Model file for the job. Use its own axes, mm. Give positions to 0.01 mm unless a question says otherwise; leave off trailing zeros. Loops run counter-clockwise (first coordinate to the right, second up) from the corner with the lowest first, then second, coordinate; pieces in that order, holes last. Notation, with made-up numbers: (-27.75, 60) - (-20.75, 60) arc R29 ccw to (-20.75, 96) - close; hole circle Ø7 at (33.5, -32.5). An arc over 180 degrees is marked (long way). Answer as CSV lines item,"result". Start each with the question number.
Item 1: Saw through at B-B on z = -81. Give the cut face in (x, y).
Item 2: Saw through at A-A on x = 0. Give the cut face in (y, z), plus the area to 3 significant figures.
Item 3: Drill centre lines: L1, parallel to Z at x = 4.75, y = 0.75; L2, parallel to Y at x = 0.25, z = -88; L3, parallel to X at y = -2.5, z = -44.5. Where is each one in solid material? Low to high. Write a range as from..to.
Item 4: Pin check, flat tips, straight feed: pin 1 (2 mm diameter, centred on y = 1, z = -64, fed in from +X); pin 2 (4 mm diameter, centred on y = 1, z = -36, fed in from -X); pin 3 (1.5 mm diameter, centred on y = -3, z = -92.5, fed in from -X). Stop position of each tip, or through.
from build123d import *

# Parameters (mm, degrees)
F0_R     = 4
F1_DEPTH = 7
F2_DEPTH = 110
F3_SIZE  = 1.5
F4_SIZE2 = 1
F4_SIZE  = 1


with BuildPart() as f1:
    # F0 (on Top) → F1 (new body)
    with BuildSketch(Plane.XY):
        Polygon((3.752777, 6.5), (-3.752777, 6.5), (-7.505553, 0), (-3.752777, -6.5), (3.752777, -6.5), (7.505553, 0), align=None)
        Circle(F0_R, mode=Mode.SUBTRACT)
        Circle(F0_R)
    extrude(amount=F1_DEPTH)

    # F0 (on Top) → F2 (join)
    with BuildSketch(Plane.XY):
        Circle(F0_R)
    extrude(amount=-F2_DEPTH)

    # F3
    f3_edges = [f1.edges().sort_by_distance(p)[0] for p in [
        (-4, 0, -110),
    ]]
    chamfer(f3_edges, length=F3_SIZE)

    # F4
    f4_edges = [f1.edges().sort_by_distance(p)[0] for p in [
        (5.629165, 3.25, 7),
        (0, 6.5, 7),
        (-5.629165, 3.25, 7),
        (-5.629165, -3.25, 7),
        (0, -6.5, 7),
        (5.629165, -3.25, 7),
    ]]
    chamfer(f4_edges, length=F4_SIZE, length2=F4_SIZE2)


solid = f1.part
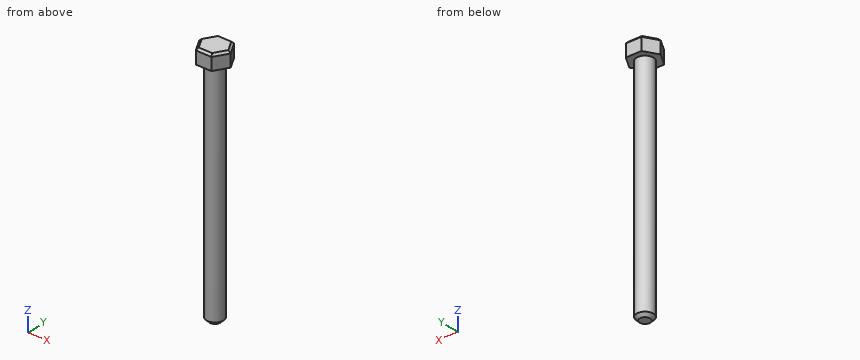
Responses:
1,outline,"circle Ø8 at (0, 0)"
2,outline,"(-6.5, 0) - (-4, 0) - (-4, -108.5) - (-2.5, -110) - (2.5, -110) - (4, -108.5) - (4, 0) - (6.5, 0) - (6.5, 6) - (5.5, 7) - (-5.5, 7) - (-6.5, 6) - close"
2,area,"968 mm2"
3,L1,"0..7"
3,L2,"-3.99..3.99"
3,L3,"-3.12..3.12"
4,pin 1,"x = 4"
4,pin 2,"x = -4"
4,pin 3,"x = -3.31"
